The model under review builds one solid part; all positions refer to its coordinate system, in mm. Face numbers are marked on the shaded views. A direction names the side the tool comes from. Round coordinates to 2 decimals unless told otherwise and drop trailing zeros. Write each loop counter-clockwise with the first axis right and the second up, starting at its lowest first coordinate (ties: lowest second). Pieces come first, ordered by that corner, then holes. Notation, with made-up numbers: M 11.25,10 L 43.25,10 A25 ccw 43.25,23 Z; hole C 70.5,55 d10. An arc over 180 degrees is marked long. One line per item, written item: value. Start each with the question number.
1) Take a section at D-D, the plane x = 21. Write out the cut boundary in (y, z), and give its area (3 significant figures).
2) Take a section at B-B, the plane y = -36.5. Write out the cut boundary in (x, z), and give its area (3 significant figures).
3) For P1, Ø1.5, axis at x = 37.5, y = -4, coming from the -Z side; P2, Ø1, axis at x = 27, y = -23, coming from the +Z side; P3, Ø3, axis at y = -20.5, z = 47.5, coming from the +X side, all flat-tipped, find the tip position at first contact; note any pin that passes through.
4) Take a section at A-A, the plane x = 5.5. Write out the cut boundary in (y, z), and give its area (3 significant figures).
5) Take a section at C-C, the plane z = 31. Write out the cut boundary in (x, y).
6) Tool access review of the marked faces 1 and 2: name each direction out of +Z, -Z, +X, -X, +Y, -Y from which nothing blocks a thin tool from reaching the whole face with its end or side.
7) Wall thickness on probe 1 along Y at (x, z) = (36.5, 27); probe 2 along X at (y, z) = (-36.5, 16.5); probe 3 along X at (y, z) = (-5, 11): over which ranges is each line inside the solid? List them lowest first.
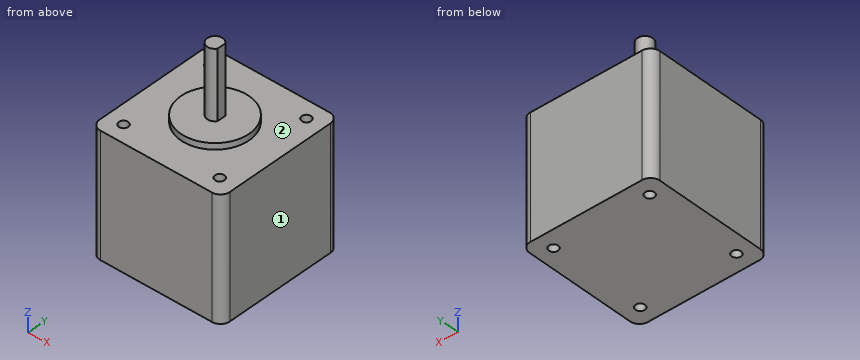
Autodesk Fusion 360 part; units mm, degrees
box "BoxPrimitive1" add length 42 width 42 height 39.3 placed x (0, -1, 0) y (1, 0, 0) z (0, 0, 1) at (0, 0, 0)
sketch "Sketch2" plane through (0, 0, 39.3) normal (0, 0, 1) x (-1, 0, 0)
  line L0 (0, 42) -> (-42, 42)
  line L1 (-42, 42) -> (-42, 0)
  line L2 (-42, 0) -> (0, 0)
  line L3 (0, 0) -> (0, 42)
  circle A0 centre (-21, 21) radius 11
  line L4 (-23.1, 22.3565) -> (-23.1, 19.6435)
  arc A1 (-23.1, 19.6435) -> (-23.1, 22.3565) centre (-21, 21) ccw
  circle A2 centre (-36.5, 36.5) radius 1.5
  circle A3 centre (-5.5, 36.5) radius 1.5
  line L5 (-5.5, 36.5) -> (-36.5, 36.5) construction
  line L6 (-36.5, 36.5) -> (-36.5, 5.5) construction
  circle A4 centre (-36.5, 5.5) radius 1.5
  circle A5 centre (-5.5, 5.5) radius 1.5
  point P0 (-21, 0)
  point P1 (0, 21)
  point P2 (-21, 36.5)
  point P3 (-21, 42)
  point P4 (-36.5, 21)
  point P5 (-42, 21)
  dimension "d8" = 22
  dimension "d11" = 5
  dimension "d14" = 2.1
  dimension "d17" = 3
  dimension "d20" = 3
  dimension "d21" = 31
  dimension "d22" = 31
  dimension "d23" = 3
  dimension "d24" = 3
extrude "Extrude2" add sketch "Sketch2" along normal blind 24 contours L4 A1
extrude "Extrude1" add sketch "Sketch2" along normal blind 2 contours A0 | L4 A1
fillet "Fillet1" radius 3 4 edges at (0, 0, 19.65) (0, -42, 19.65) (42, -42, 19.65) (42, 0, 19.65)
extrude "Extrude3" cut sketch "Sketch2" against normal blind 40 contours A2 | A3 | A4 | A5
Checked values:
1. outline: M -42,0 L 0,0 L 0,39.3 L -10,39.3 L -10,41.3 L -18.5,41.3 L -18.5,63.3 L -23.5,63.3 L -23.5,41.3 L -32,41.3 L -32,39.3 L -42,39.3 Z
1. area: 1,800 mm2
2. outline: M 0,0 L 4,0 L 4,39.3 L 0,39.3 Z; M 7,0 L 35,0 L 35,39.3 L 7,39.3 Z; M 38,0 L 42,0 L 42,39.3 L 38,39.3 Z
2. area: 1,410 mm2
3. P1: stops at z = 0
3. P2: stops at z = 41.3
3. P3: stops at x = 23.1
4. outline: M -42,0 L -38,0 L -38,39.3 L -42,39.3 Z; M -35,0 L -7,0 L -7,39.3 L -35,39.3 Z; M -4,0 L 0,0 L 0,39.3 L -4,39.3 Z
4. area: 1,410 mm2
5. outline: M 0,-39 A3 ccw 3,-42 L 39,-42 A3 ccw 42,-39 L 42,-3 A3 ccw 39,0 L 3,0 A3 ccw 0,-3 Z; hole C 5.5,-36.5 d3; hole C 5.5,-5.5 d3; hole C 36.5,-36.5 d3; hole C 36.5,-5.5 d3
6. face 1: +Z, -Z, +X, +Y, -Y
6. face 2: +Z
7. probe 1: y = -42 to -38, -35 to -7, -4 to 0
7. probe 2: x = 0 to 4, 7 to 35, 38 to 42
7. probe 3: x = 0 to 4.09, 6.91 to 35.09, 37.91 to 42
